For this review, use the dimensioned drawing (mm, ordinates from the lowest corner) and the shaded views. A direction names the side the tool comes from. Give positions to 0.01 mm unless a question says otherwise; leave off trailing zeros. Order: outer loops, then holes, each group sorted by start corner. A loop starts at its lowest first (then second) coordinate and runs counter-clockwise, first axis right, second up. Notation, with made-up numbers: (0.25, -19) -> (52.25, -19) arc R11 cw to (52.25, -12) -> close; hole circle Ø7 at (29, 50). An arc over 180 degrees is marked (long way). Answer as a JSON object with one key per item and string values. Group by question number.
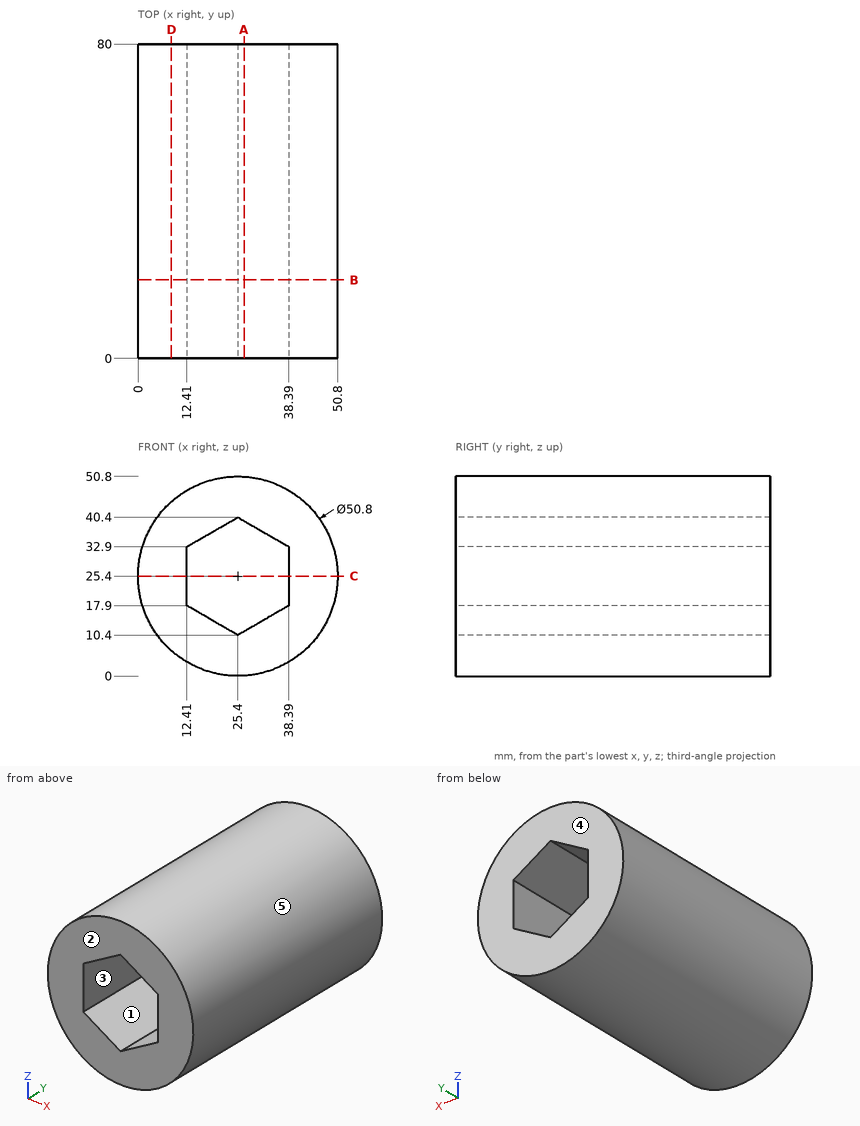
1. For pin 1 (1 mm diameter, centred on x = 38.5, z = 22, fed in from -Y); pin 2 (8 mm diameter, centred on x = 18.5, y = 32.5, fed in from -Z); pin 3 (2 mm diameter, centred on x = 30, y = 53.5, fed in from +Z); pin 4 (8 mm diameter, centred on x = 27.5, z = 31.5, fed in from -Y), all flat-tipped, find the tip position at first contact; note any pin that passes through.
2. Draft analysis for pull direction X (two halves, no side actions). For the marked faces 3, 4 and 5, state which applies: pulls with the +X half, pulls with the -X half, needs draft (parallel to the pull), parting line crosses it, or undercut.
3. Take a section at C-C on z = 25.4. Give the boundary of the cut face in (x, y), plus the area to 3 significant figures.
4. Take a section at B-B on y = 20. Give the boundary of the cut face in (x, z).
5. Take a section at D-D on x = 8.5. Give the boundary of the cut face in (y, z), plus the area to 3 significant figures.
6. Take a section at A-A on x = 27. Give the boundary of the cut face in (y, z).
7. Machinability: for the marked faces 1 and 2, which of the approach directions +Z, -Z, +X, -X, +Y, -Y give a long, thin tool a straight path to every point of the face, cutting with its end or side? Answer none if there is none.
8. For probe 1 along X at (y, z) = (28, 13.5); probe 2 along Z at (x, y) = (26, 66.5) (1 decimal); probe 3 along Z at (x, y) = (36, 11), list the stretches that pass through material, from the lowest coordinate up. Write a range as [from, to].
Checks:
{
 "1": {"pin 1": "stops at y = 0", "pin 2": "stops at z = 0.17", "pin 3": "stops at z = 50.54", "pin 4": "passes through"},
 "2": {"face 3": "undercut", "face 4": "needs draft", "face 5": "parting line crosses it"},
 "3": {"outline": "(0, 0) -> (12.41, 0) -> (12.41, 80) -> (0, 80) -> close; (38.39, 0) -> (50.8, 0) -> (50.8, 80) -> (38.39, 80) -> close", "area": "1,990 mm2"},
 "4": {"outline": "circle Ø50.8 at (25.4, 25.4); hole (12.41, 17.9) -> (25.4, 10.4) -> (38.39, 17.9) -> (38.39, 32.9) -> (25.4, 40.4) -> (12.41, 32.9) -> close"},
 "5": {"outline": "(0, 6.44) -> (80, 6.44) -> (80, 44.36) -> (0, 44.36) -> close", "area": "3,030 mm2"},
 "6": {"outline": "(0, 0.05) -> (80, 0.05) -> (80, 11.32) -> (0, 11.32) -> close; (0, 39.48) -> (80, 39.48) -> (80, 50.75) -> (0, 50.75) -> close"},
 "7": {"face 1": "+Y, -Y", "face 2": "+Z, -Z, +X, -X, -Y"},
 "8": {"probe 1": "x = [2.96, 20.03], [30.77, 47.84]", "probe 2": "z = [0, 10.7], [40.1, 50.8]", "probe 3": "z = [2.32, 16.52], [34.28, 48.48]"}
}
